Autodesk Inventor part; units mm, degrees
ref_plane "YZ Plane" through (0, 0, 0) normal (1, 0, 0) x (0, 1, 0)
ref_plane "XZ Plane" through (0, 0, 0) normal (0, 1, 0) x (-1, 0, 0)
ref_plane "XY Plane" through (0, 0, 0) normal (0, 0, 1) x (1, 0, 0)
sketch "Sketch1" plane through (0, 0, 0) normal (0, 0, 1) x (1, 0, 0)
  line L0 (7, -20) -> (7, -17)
  line L1 (-7, -17) -> (7, -17)
  line L2 (-7, -17) -> (-7, -20)
  arc A0 (-7, -20) -> (-4.5, -22.5) centre (-4.5, -20) ccw
  line L3 (-4.5, -22.5) -> (4.5, -22.5)
  arc A1 (4.5, -22.5) -> (7, -20) centre (4.5, -20) ccw
  circle A2 centre (-4.5, -20) radius 1
  circle A3 centre (4.5, -20) radius 1
  line L4 (7, -11.4) -> (-7, -11.4)
  line L5 (-7, -11.4) -> (-7, -17)
  line L6 (-7, -17) -> (7, -17)
  line L7 (7, -17) -> (7, -11.4)
  circle A4 centre (4.5, -14.2) radius 0.9
  circle A5 centre (-4.5, -14.2) radius 0.9
  point P0 (0, 0)
extrude "Extrusion1" add sketch "Sketch1" along normal blind 3
sketch "Sketch2" plane through (0, 0, 3) normal (0, 0, 1) x (1, 0, 0)
  circle A0 centre (-4.5, -20) radius 1
  circle A1 centre (4.5, -20) radius 1
  circle A2 centre (0, -27.2111) radius 6.5
  point P0 (0, 0)
extrude "Extrusion2" cut sketch "Sketch2" against normal blind 3 contours A2
fillet "Fillet1" radius 1 2 edges at (-4.4783, -22.5, 1.5) (4.4783, -22.5, 1.5)
properties part number "upper slider pen"
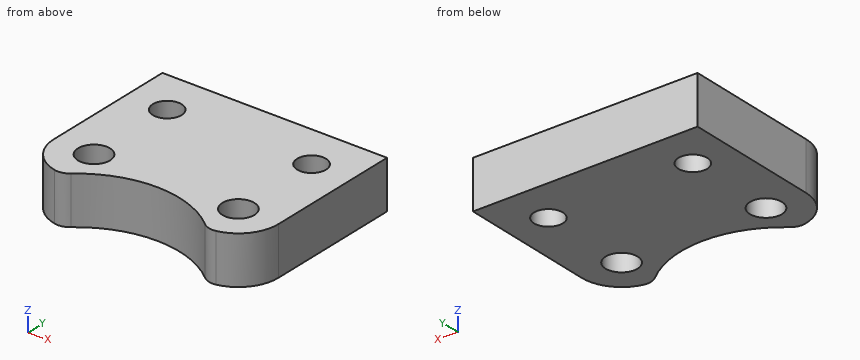
The model under review builds one solid part; all positions refer to its coordinate system, in mm. Round coordinates to 2 decimals unless told otherwise and drop trailing zeros. Order: outer loops, then holes, each group sorted by start corner. A loop starts at its lowest first (then second) coordinate and runs counter-clockwise, first axis right, second up.
Item 1: Add section C-C, the plane y = -20.5. State the section outline as (x, z) points, and give its area (3 significant figures).
Working result:
outline: (-6.95, 0) - (-5.37, 0) - (-5.37, 3) - (-6.95, 3) - close; (-3.63, 0) - (3.63, 0) - (3.63, 3) - (-3.63, 3) - close; (5.37, 0) - (6.95, 0) - (6.95, 3) - (5.37, 3) - close
area: 31.3 mm2
Item 2: For pin 1 (1.2 mm diameter, centred on x = -4.5, y = -20, fed in from -Z); pin 2 (2.5 mm diameter, centred on x = 4.5, y = -14.2, fed in from +Z), all flat-tipped, find the tip position at first contact; note any pin that passes through.
Working result:
pin 1: passes through
pin 2: stops at z = 3
Item 3: Add section B-B, the plane z = 0.2. Count the separate pieces of the cut face and the enclosed holes in it, and give its area (3 significant figures).
Working result:
separate pieces: 1
enclosed holes: 4
area: 130 mm2
Item 4: Add section D-D, the plane x = 0. State the section outline as (y, z) points, and give its area (3 significant figures).
Working result:
outline: (-20.71, 0) - (-11.4, 0) - (-11.4, 3) - (-20.71, 3) - close
area: 27.9 mm2
Item 5: To check wall thickness, follow probe 1 along Y at (x, z) = (4.5, 2.05); probe 2 along Y at (x, z) = (-5, 1.9); probe 3 along X at (y, z) = (-13.5, 2.3). State the ranges of each line that lie inside material, in increasing order.
Working result:
probe 1: y = -22.41 to -21, -19 to -15.1, -13.3 to -11.4
probe 2: y = -22.45 to -20.87, -19.13 to -14.95, -13.45 to -11.4
probe 3: x = -7 to -5.07, -3.93 to 3.93, 5.07 to 7
Item 6: Add section A-A, the plane y = -14.2. State the section outline as (x, z) points, and give its area (3 significant figures).
Working result:
outline: (-7, 0) - (-5.4, 0) - (-5.4, 3) - (-7, 3) - close; (-3.6, 0) - (3.6, 0) - (3.6, 3) - (-3.6, 3) - close; (5.4, 0) - (7, 0) - (7, 3) - (5.4, 3) - close
area: 31.2 mm2
